Source: three-view drawing plus pictorial views. Frame: mm from the lowest corner of the part. A direction names the side the tool comes from. Coordinates: 2 decimals unless noted, no trailing zeros. Order: outer loops, then holes, each group sorted by start corner. A loop starts at its lowest first (then second) coordinate and runs counter-clockwise, first axis right, second up. Notation, with made-up numbers: (-0.75, 37.25) - (31.25, 37.25) arc R9 ccw to (31.25, 46.25) - close; hole circle Ø3 at (-11, 53.5). An arc over 180 degrees is marked (long way). Use a Markdown table: item, result. Add a question column.
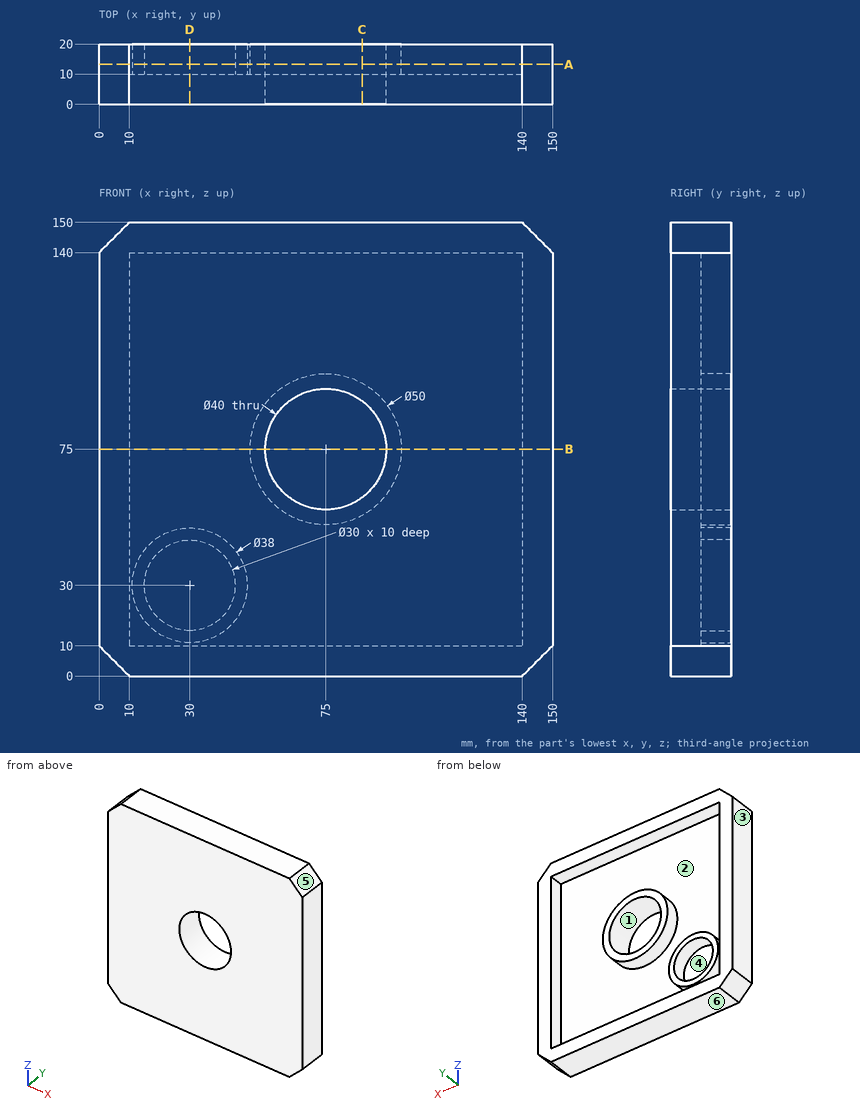
1) Section D-D (x = 30). Return loops of the section in (y, z).
2) Pin query (flat end, axial travel): pin 1 (15 mm diameter, centred on x = 30.5, z = 29.5, fed in from +Y). Return the tip coordinate at first contact, or that it passes through.
3) Ray query, line 1 along X through (y, z) = (15, 30); line 2 along X through (y, z) = (11, 75); line 3 along X through (y, z) = (12.75, 111). Return the intervals inside material, ascending.
4) Set-up query: the marked faces 1 and 2. Return all of +Z, -Z, +X, -X, +Y, -Y with unobstructed straight access to the full face (end or side cutting, diameter ignored); none if empty.
5) Section C-C (x = 87). Return loops of the section in (y, z).
6) Draft query along Z for the marked faces 3, 4, 5 and 6. Return one class per face: pulls with the +Z half, pulls with the -Z half, needs draft (parallel to the pull), parting line crosses it, or undercut.
7) Section A-A (y = 13.25). Return loops of the section in (x, z), then the cut area to 3 significant figures.
8) Section B-B (z = 75). Return loops of the section in (x, y).
Values follow:
| question | item | result |
|---|---|---|
| 1 | outline | (0, 0) - (20, 0) - (20, 10) - (10, 10) - (10, 11) - (20, 11) - (20, 15) - (10, 15) - (10, 45) - (20, 45) - (20, 49) - (10, 49) - (10, 140) - (20, 140) - (20, 150) - (0, 150) - close |
| 2 | pin 1 | stops at y = 10 |
| 3 | line 1 | x = 0 to 10, 11 to 15, 45 to 49, 140 to 150 |
| 3 | line 2 | x = 0 to 10, 50 to 55, 95 to 100, 140 to 150 |
| 3 | line 3 | x = 0 to 10, 140 to 150 |
| 4 | face 1 | +Y, -Y |
| 4 | face 2 | +Y |
| 5 | outline | (0, 0) - (20, 0) - (20, 10) - (10, 10) - (10, 53.07) - (20, 53.07) - (20, 59) - (0, 59) - close; (0, 91) - (20, 91) - (20, 96.93) - (10, 96.93) - (10, 140) - (20, 140) - (20, 150) - (0, 150) - close |
| 6 | face 3 | needs draft |
| 6 | face 4 | undercut |
| 6 | face 5 | pulls with the +Z half |
| 6 | face 6 | pulls with the -Z half |
| 7 | outline | (0, 10) - (10, 0) - (140, 0) - (150, 10) - (150, 140) - (140, 150) - (10, 150) - (0, 140) - close; circle Ø38 at (30, 30); circle Ø50 at (75, 75); hole (10, 10) - (140, 10) - (140, 140) - (10, 140) - close; hole circle Ø30 at (30, 30); hole circle Ø40 at (75, 75) |
| 7 | area | 6,530 mm² |
| 8 | outline | (0, 0) - (55, 0) - (55, 20) - (50, 20) - (50, 10) - (10, 10) - (10, 20) - (0, 20) - close; (95, 0) - (150, 0) - (150, 20) - (140, 20) - (140, 10) - (100, 10) - (100, 20) - (95, 20) - close |
